Design review of the part shown in the three views and the two pictorial views. Dimensions are in mm from the part's minimum x, y and z. A direction names the side the tool comes from. Coordinates: 2 decimals unless noted, no trailing zeros. Order: outer loops, then holes, each group sorted by start corner. A loop starts at its lowest first (then second) coordinate and runs counter-clockwise, first axis right, second up. Notation, with made-up numbers: (-25.75, 51.5) -> (-4.75, 51.5) arc R36 cw to (-4.75, 87.5) -> close; hole circle Ø10 at (-40, -11). An arc over 180 degrees is marked (long way). Answer as a JSON object with one key per item and string values. Group by question number.
1) Machinability: for the marked faces 4, 5 and 6, which of the approach directions +Z, -Z, +X, -X, +Y, -Y give a long, thin tool a straight path to every point of the face, cutting with its end or side? Answer none if there is none.
2) Add section D-D, the plane y = 13.5. Write out the cut boundary in (x, z).
3) Add section A-A, the plane y = 7.5. Write out the cut boundary in (x, z), then the cut area to 3 significant figures.
4) Add section C-C, the plane x = 15.25. Write out the cut boundary in (y, z).
5) For pin 1 (5 mm diameter, centred on x = 11, z = 4.5, fed in from -Y); pin 2 (6 mm diameter, centred on x = 16, y = 13, fed in from -Z); pin 3 (4 mm diameter, centred on x = 13.5, y = 5, fed in from -Z); pin 4 (9 mm diameter, centred on y = 6.5, z = 9, fed in from -X), all flat-tipped, find the tip position at first contact; note any pin that passes through.
6) Draft analysis for pull direction X (two halves, no side actions). For the marked faces 1, 2 and 3, state which applies: +X half, -X half, draft (parallel to the pull), parting line (faces both ways), or undercut.
7) Wall thickness on L1, parallel to X at y = 11.75, z = 12.5; L2, parallel to Z at x = 5.75, y = 5.5; L3, parallel to Z at x = 18, y = 10: over which ranges is each line inside the solid? List them lowest first.
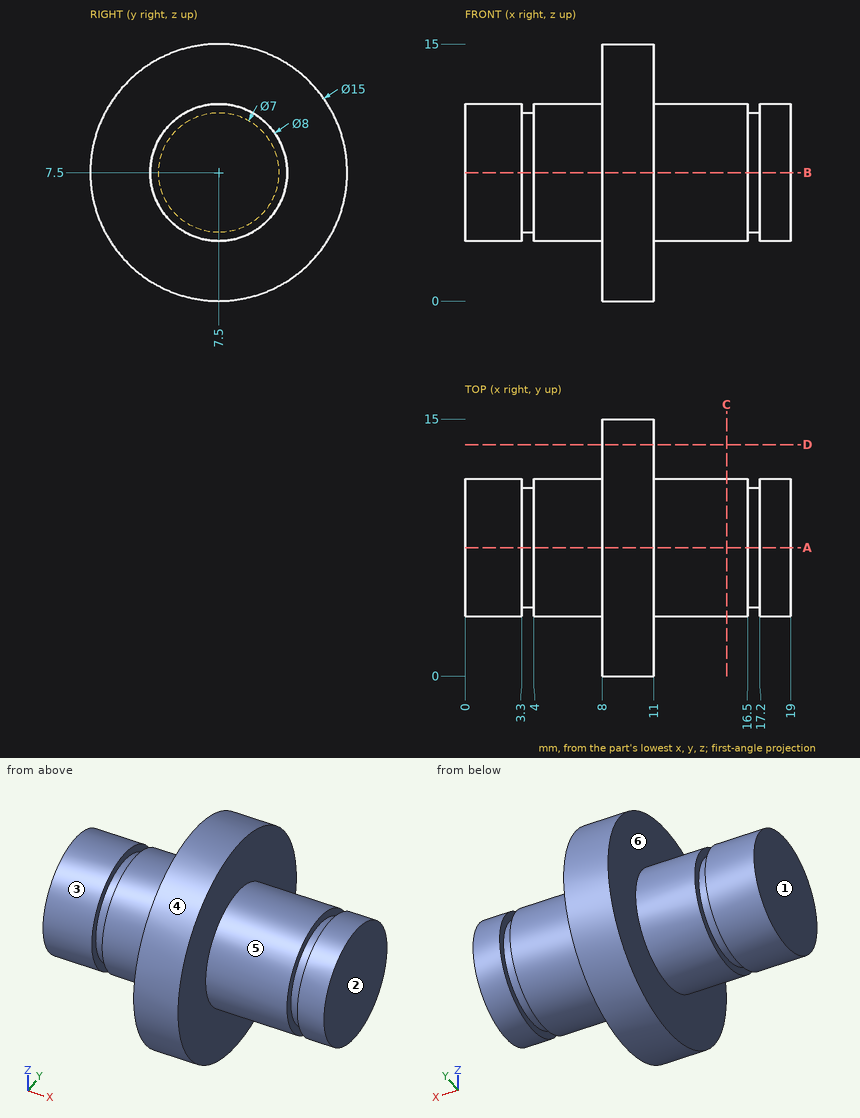
Output values:
{
 "1": {"face 4": "+X, -X", "face 5": "+X", "face 6": "-X"},
 "2": {"outline": "(8, 3) -> (11, 3) -> (11, 12) -> (8, 12) -> close"},
 "3": {"outline": "(0, 3.5) -> (3.3, 3.5) -> (3.3, 4) -> (4, 4) -> (4, 3.5) -> (8, 3.5) -> (8, 0) -> (11, 0) -> (11, 3.5) -> (16.5, 3.5) -> (16.5, 4) -> (17.2, 4) -> (17.2, 3.5) -> (19, 3.5) -> (19, 11.5) -> (17.2, 11.5) -> (17.2, 11) -> (16.5, 11) -> (16.5, 11.5) -> (11, 11.5) -> (11, 15) -> (8, 15) -> (8, 11.5) -> (4, 11.5) -> (4, 11) -> (3.3, 11) -> (3.3, 11.5) -> (0, 11.5) -> close", "area": "172 mm²"},
 "4": {"outline": "circle Ø8 at (7.5, 7.5)"},
 "5": {"pin 1": "stops at y = 0.02", "pin 2": "stops at z = 4.38", "pin 3": "stops at z = 3.53", "pin 4": "stops at x = 0"},
 "6": {"face 1": "-X half", "face 2": "+X half", "face 3": "draft"},
 "7": {"L1": "x = 8 to 11", "L2": "z = 4.04 to 10.96", "L3": "z = 4.38 to 10.62"}
}
